Check sheet for the modelled part. Datum: model origin and axes. Units: mm. Face numbers are marked on the shaded views. A direction names the side the tool comes from. Round coordinates to 2 decimals unless told otherwise and drop trailing zeros. Loops run counter-clockwise (first coordinate to the right, second up) from the corner with the lowest first, then second, coordinate; pieces in that order, holes last. Notation, with made-up numbers: (27.25, 3.5) -> (37.25, 3.5) arc R30 ccw to (37.25, 37.5) -> close; hole circle Ø4 at (70.5, 5.5). An arc over 180 degrees is marked (long way). One line per question, with ' | ' between items.
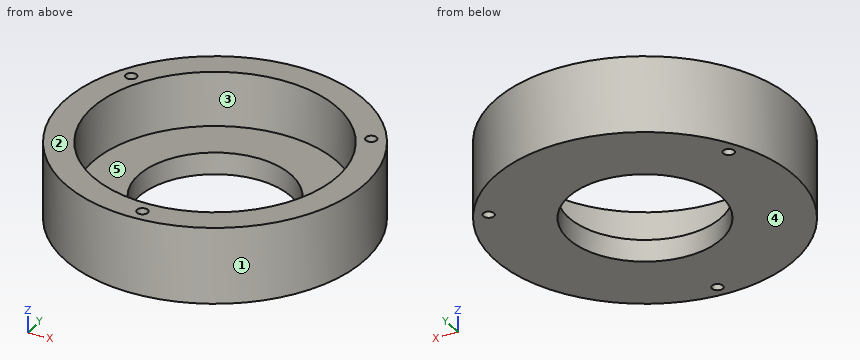
```python
from build123d import *

# Parameters (mm, degrees)
SKETCH_R      = 27.5
SKETCH_R_2    = 14
PAD_DEPTH     = 4
SKETCH005_R   = 27.5
SKETCH005_R_2 = 22.5
PAD001_DEPTH  = 10
SKETCH006_R   = 1
POCKET_DEPTH  = 14.001


with BuildPart() as part:
    # Sketch → Pad (new body)
    with BuildSketch(Plane.XY):
        Circle(SKETCH_R)
        Circle(SKETCH_R_2, mode=Mode.SUBTRACT)
    extrude(amount=PAD_DEPTH)

    # Sketch005 (on Face4 of Pad) → Pad001 (join)
    with BuildSketch(Plane.XY.offset(4)):
        Circle(SKETCH005_R)
        Circle(SKETCH005_R_2, mode=Mode.SUBTRACT)
    extrude(amount=PAD001_DEPTH)

    # Sketch006 (on Face2 of Pad001) → Pocket (cut, through all)
    with BuildSketch(Plane(origin=(0, 0, 0), x_dir=(1, 0, 0), z_dir=(0, 0, -1))):
        with Locations((0, 25)):
            Circle(SKETCH006_R)
        with Locations((-21.650635, -12.5)):
            Circle(SKETCH006_R)
        with Locations((21.650635, -12.5)):
            Circle(SKETCH006_R)
    extrude(amount=-POCKET_DEPTH, mode=Mode.SUBTRACT)


solid = part.part
```
(1) Go/stop test with flat-tipped pins: pin 1 (2 mm diameter, centred on y = -8.5, z = 8, fed in from -X); pin 2 (1.8 mm diameter, centred on x = 0, y = -25, fed in from +Z); pin 3 (2 mm diameter, centred on x = -19.5, z = 11, fed in from +Y); pin 4 (5 mm diameter, centred on y = -7.5, z = 11, fed in from +X). Record where each tip stops, or that it passes through.
Answer:
pin 1: stops at x = -26.46 | pin 2: passes through | pin 3: stops at y = 20.35 | pin 4: stops at x = 27.04
(2) Sectioned sample at A-A, the plane x = 0. Record the cut outline in (y, z), and give its area (3 significant figures).
Answer:
outline: (-27.5, 0) -> (-26, 0) -> (-26, 14) -> (-27.5, 14) -> close; (-24, 0) -> (-14, 0) -> (-14, 4) -> (-22.5, 4) -> (-22.5, 14) -> (-24, 14) -> close; (14, 0) -> (27.5, 0) -> (27.5, 14) -> (22.5, 14) -> (22.5, 4) -> (14, 4) -> close | area: 180 mm2
(3) Mould release check, pull along Y, two halves, no side actions. Record for the marked faces 1, 2 and 3: +Y half, -Y half, draft (parallel to the pull), parting line (faces both ways), or undercut.
Answer:
face 1: parting line | face 2: draft | face 3: undercut
(4) Sectioned sample at B-B, the plane y = 0. Record the cut outline in (x, z).
Answer:
outline: (-27.5, 0) -> (-14, 0) -> (-14, 4) -> (-22.5, 4) -> (-22.5, 14) -> (-27.5, 14) -> close; (14, 0) -> (27.5, 0) -> (27.5, 14) -> (22.5, 14) -> (22.5, 4) -> (14, 4) -> close
(5) Sectioned sample at D-D, the plane x = -8. Record the cut outline in (y, z), and give its area (3 significant figures).
Answer:
outline: (-26.31, 0) -> (-11.49, 0) -> (-11.49, 4) -> (-21.03, 4) -> (-21.03, 14) -> (-26.31, 14) -> close; (11.49, 0) -> (26.31, 0) -> (26.31, 14) -> (21.03, 14) -> (21.03, 4) -> (11.49, 4) -> close | area: 224 mm2
(6) Scan lines: probe 1 along Y at (x, z) = (0, 2); probe 2 along Y at (x, z) = (0, 9); probe 3 along Z at (x, y) = (-4.5, 15). Record each from-to range of solid material in increasing order.
Answer:
probe 1: y = -27.5 to -26, -24 to -14, 14 to 27.5 | probe 2: y = -27.5 to -26, -24 to -22.5, 22.5 to 27.5 | probe 3: z = 0 to 4
(7) Sectioned sample at C-C, the plane y = 12.5. Record the cut outline in (x, z).
Answer:
outline: (-24.49, 0) -> (-22.65, 0) -> (-22.65, 14) -> (-24.49, 14) -> close; (-20.65, 0) -> (-6.3, 0) -> (-6.3, 4) -> (-18.71, 4) -> (-18.71, 14) -> (-20.65, 14) -> close; (6.3, 0) -> (20.65, 0) -> (20.65, 14) -> (18.71, 14) -> (18.71, 4) -> (6.3, 4) -> close; (22.65, 0) -> (24.49, 0) -> (24.49, 14) -> (22.65, 14) -> close
(8) Set-up check for the marked faces 4 and 5: record each of +Z, -Z, +X, -X, +Y, -Y from which the full face is reachable in a straight line by a thin tool's end or side.
Answer:
face 4: -Z, +X, -X, +Y, -Y | face 5: +Z
